from build123d import *

# Parameters (mm, degrees)
F0_R     = 41.14767
F1_DEPTH = 158.304572
F2_W     = 30.046224
F2_H     = 18.724471
F3_DEPTH = 635
F4_W     = 39.408475
F4_H     = 19.81309
F5_DEPTH = 63.5
F6_R     = 32.223353
F7_DEPTH = 25.4


with BuildPart() as f1:
    # F0 (on Top) → F1 (new body)
    with BuildSketch(Plane.XY):
        Circle(F0_R)
    extrude(amount=F1_DEPTH)

    # F2 (on Front) → F3 (cut, symmetric)
    with BuildSketch(Plane.XZ):
        with Locations((32.005787, 76.323956)):
            Rectangle(F2_W, F2_H)
    extrude(amount=F3_DEPTH, both=True, mode=Mode.SUBTRACT)

    # F4 (on Front) → F5 (cut, symmetric)
    with BuildSketch(Plane.XZ):
        with Locations((-31.679184, 74.255556)):
            Rectangle(F4_W, F4_H)
    extrude(amount=F5_DEPTH, both=True, mode=Mode.SUBTRACT)

    # F6 (on face) → F7 (join)
    with BuildSketch(Plane.XY.offset(158.304572)):
        Circle(F6_R)
    extrude(amount=F7_DEPTH)


solid = f1.part
Build history of the part. All positions in model axes, mm. A direction names the side the tool comes from. Coordinates: 2 decimals unless noted, no trailing zeros. Write each loop counter-clockwise with the first axis right and the second up, starting at its lowest first coordinate (ties: lowest second). Pieces come first, ordered by that corner, then holes.
(1) Cut at D-D on z = 165.5. List the corners of the cut face in (x, y), and give its area (3 significant figures).
(2) Cut at C-C on x = 28. List the corners of the cut face in (y, z), and give its area (3 significant figures).
(3) Cut at A-A on y = 0. List the corners of the cut face in (x, z), and give its area (3 significant figures).
(4) Cut at B-B on x = 0. List the corners of the cut face in (y, z).
(5) Drill centre lines: line 1 (Z direction, x = -31, y = 16); line 2 (Z direction, x = 32, y = 18); line 3 (X direction, y = 1.5, z = 154). Where is each one in solid material? Low to high.
(6) 3-axis set-ups, long thin cutter, end or side, ignore diameter. For faces 4 (the flat face through (-11.975, -1, 74)), 5 (the flat face through (26, -1, 66.962)), 6 (the cylindrical face through (-8.92, -40.17, 78.04)), 7 (the flat face through (-25, -21, 158.305)): which of +Z, -Z, +X, -X, +Y, -Y reach the whole face in a straight line?
(7) Pin check, flat tips, straight feed: pin 1 Ø20.5 at (y, z) = (12, 72) entering from +X; pin 2 Ø10 at (y, z) = (-28, 111) entering from -X; pin 3 Ø3 at (y, z) = (-14, 19.5) entering from -X. Stop position of each tip, or through.
(8) Mould opens along Z. For faces 1 (the flat face through (-24, -1, 64.349)), 2 (the flat face through (-1, 1, 0)), 3 (the flat face through (0, 0, 183.705)) say: pulls with the +Z half, pulls with the -Z half, needs draft (parallel to the pull), parting line crosses it, or undercut.
Working result:
1. outline: circle Ø64.45 at (0, 0)
1. area: 3,260 mm2
2. outline: (-30.15, 0) - (30.15, 0) - (30.15, 66.96) - (-30.15, 66.96) - close; (-30.15, 85.69) - (30.15, 85.69) - (30.15, 158.3) - (15.95, 158.3) - (15.95, 183.7) - (-15.95, 183.7) - (-15.95, 158.3) - (-30.15, 158.3) - close
2. area: 9,230 mm2
3. outline: (-41.15, 0) - (41.15, 0) - (41.15, 66.96) - (16.98, 66.96) - (16.98, 85.69) - (41.15, 85.69) - (41.15, 158.3) - (32.22, 158.3) - (32.22, 183.7) - (-32.22, 183.7) - (-32.22, 158.3) - (-41.15, 158.3) - (-41.15, 84.16) - (-11.97, 84.16) - (-11.97, 64.35) - (-41.15, 64.35) - close
3. area: 13,600 mm2
4. outline: (-41.15, 0) - (41.15, 0) - (41.15, 158.3) - (32.22, 158.3) - (32.22, 183.7) - (-32.22, 183.7) - (-32.22, 158.3) - (-41.15, 158.3) - close
5. line 1: z = 0 to 64.35, 84.16 to 158.3
5. line 2: z = 0 to 66.96, 85.69 to 158.3
5. line 3: x = -41.12 to 41.12
6. face 4: -X, +Y, -Y
6. face 5: +X, +Y, -Y
6. face 6: +Z, -Z
6. face 7: +Z
7. pin 1: stops at x = 41.03
7. pin 2: stops at x = -34.12
7. pin 3: stops at x = -39.2
8. face 1: undercut
8. face 2: pulls with the -Z half
8. face 3: pulls with the +Z half
